Check sheet for the modelled part. Datum: model origin and axes. Units: mm. A direction names the side the tool comes from. Round coordinates to 2 decimals unless told otherwise and drop trailing zeros. Order: outer loops, then holes, each group sorted by start corner. A loop starts at its lowest first (then second) coordinate and runs counter-clockwise, first axis right, second up. Notation, with made-up numbers: M 26,59.25 L 32,59.25 A7 cw 32,63.25 Z; hole C 60.25,51.5 d10. An arc over 180 degrees is marked long. One line per item, written item: value. Start each with the question number.
(1) Depth check by flat-ended pin: pin 1 Ø1.5 at (y, z) = (10.5, 0.5) entering from +X; pin 2 Ø0.7 at (y, z) = (21.5, 0.5) entering from -X; pin 3 Ø1.6 at (y, z) = (22, 0.5) entering from +X; pin 4 Ø0.8 at (x, z) = (-0.5, -0.5) entering from +Y. Enter the tip coordinate at first touch or a pass-through.
(2) Thickness scan on L1, parallel to Y at x = 2, z = -1 (3 decimals); L2, parallel to Z at x = 0.05, y = 9; L3, parallel to X at y = 21.5, z = 1. Record the ranges inside material, lowest first.
(3) Cross-section at D-D, the plane x = -2.15. Enter the section's corners in (y, z) (3 decimals), and give its area (3 significant figures).
(4) Cross-section at A-A, the plane z = 0. Enter the section's corners in (x, y) (3 decimals), and give its area (3 significant figures).
(5) Cross-section at B-B, the plane x = -0.7. Enter the section's corners in (y, z) (3 decimals).
(6) Release check for a two-part mould opening along X. For faces 1 (the face through (0.644, 21.982, 1.095)), 2 (the face through (-0.54, 21.19, -2.44)), 3 (the face through (2, 19.685, 0)) record: released by +X, released by -X, zero draft, split by the parting line, or undercut.
(7) Cross-section at C-C, the plane y = 7. Enter the section's corners in (x, z), and give its area (3 significant figures).
(8) Access from +Z, -Z, +X, -X, +Y, -Y to the whole of each face (thin tool, end or side, straight path). Record for faces 4 (the face through (1.27, 22, 0)), 5 (the face through (0, 0, 0)), 6 (the face through (1.5, 9.7, -0.07)).
Autodesk Inventor part; units mm, degrees
ref_plane "YZ Plane" through (0, 0, 0) normal (1, 0, 0) x (0, 1, 0)
ref_plane "XZ Plane" through (0, 0, 0) normal (0, 1, 0) x (-1, 0, 0)
ref_plane "XY Plane" through (0, 0, 0) normal (0, 0, 1) x (1, 0, 0)
sketch "Sketch1" plane through (0, 0, 0) normal (0, 1, 0) x (-1, 0, 0)
  circle A0 centre (0, 0) radius 1.5
  dimension "d0" = 3
extrude "Extrusion1" add sketch "Sketch1" along normal blind 19.685
sketch "Sketch2" plane through (0, 19.685, 0) normal (0, 1, 0) x (1, 0, 0)
  circle A0 centre (0, 0) radius 1.5
  circle A1 centre (0, 0) radius 2.5
  dimension "d3" = 5
extrude "Extrusion2" add sketch "Sketch2" along normal blind 3.048 contours A0 | A1
sketch "Sketch3" plane through (0, 22.733, 0) normal (0, 1, 0) x (1, 0, 0)
  circle A0 centre (0, 0) radius 2.5
  line L0 (-1.27, 0.7332) -> (0, 1.4665)
  line L1 (0, 1.4665) -> (1.27, 0.7332)
  line L2 (1.27, 0.7332) -> (1.27, -0.7332)
  line L3 (1.27, -0.7332) -> (0, -1.4665)
  line L4 (0, -1.4665) -> (-1.27, -0.7332)
  line L5 (-1.27, -0.7332) -> (-1.27, 0.7332)
  dimension "d6" = 1.27
extrude "Extrusion3" cut sketch "Sketch3" against normal blind 1.524 contours L0 L1 L2 L3 L4 L5
thread "Thread1"
properties part number "Threaded Rod Screw"
Values found:
1. pin 1: x = 1.5
1. pin 2: x = -2.5
1. pin 3: x = 2.5
1. pin 4: y = 21.21
2. L1: 19.685 to 22.733
2. L2: -1.5 to 1.5
2. L3: -2.29 to -0.81, 0.81 to 2.29
3. outline: M 19.685,-1.276 L 22.733,-1.276 L 22.733,1.276 L 19.685,1.276 Z
3. area: 7.78 mm^2
4. outline: M -2.5,19.685 L -1.5,19.685 L -1.5,0 L 1.5,0 L 1.5,19.685 L 2.5,19.685 L 2.5,22.733 L 1.27,22.733 L 1.27,21.209 L -1.27,21.209 L -1.27,22.733 L -2.5,22.733 Z
4. area: 70.4 mm^2
5. outline: M 0,-1.327 L 19.685,-1.327 L 19.685,-2.4 L 22.733,-2.4 L 22.733,-1.062 L 21.209,-1.062 L 21.209,1.062 L 22.733,1.062 L 22.733,2.4 L 19.685,2.4 L 19.685,1.327 L 0,1.327 Z
6. face 1: undercut
6. face 2: split by the parting line
6. face 3: zero draft
7. outline: C 0,0 d3
7. area: 7.07 mm^2
8. face 4: +Y
8. face 5: +Z, -Z, +X, -X, -Y
8. face 6: -Y
